from build123d import *

# Parameters (mm, degrees)
SKETCH1_R           = 1.5
BOSS_EXTRUDE1_DEPTH = 2.5
SKETCH2_R           = 2.5
BOSS_EXTRUDE2_DEPTH = 2
SKETCH3_R           = 1.49
CUT_EXTRUDE1_DEPTH  = 7


with BuildPart() as part:
    # Sketch1 → Boss-Extrude1 (new body)
    with BuildSketch(Plane(origin=(0, 0, 0), x_dir=(1, 0, 0), z_dir=(0, 1, 0))):
        with BuildLine():
            Line((-8.75, 14.25), (3.8, 14.25))
            Line((3.8, 14.25), (3.8, -14.25))
            Line((3.8, -14.25), (-8.75, -14.25))
            ThreePointArc((-8.75, -14.25), (-12.5, -18), (-8.75, -21.75))
            Line((-8.75, -21.75), (7.55, -21.75))
            ThreePointArc((7.55, -21.75), (10.201650429, -20.651650429), (11.3, -18))
            Line((11.3, -18), (11.3, 18))
            ThreePointArc((11.3, 18), (10.201650429, 20.651650429), (7.55, 21.75))
            Line((7.55, 21.75), (-8.75, 21.75))
            ThreePointArc((-8.75, 21.75), (-12.5, 18), (-8.75, 14.25))
        make_face()
        with Locations(Location((0, 18, 0), (0, 0, 270))):
            Circle(SKETCH1_R, mode=Mode.SUBTRACT)
        with Locations(Location((0, -18, 0), (0, 0, 270))):
            Circle(SKETCH1_R, mode=Mode.SUBTRACT)
    extrude(amount=BOSS_EXTRUDE1_DEPTH)

    # Sketch2 → Boss-Extrude2 (add)
    with BuildSketch(Plane.XZ):
        with Locations(Location((7.55, 0, 0), (0, 0, 90))):
            Circle(SKETCH2_R)
    extrude(amount=BOSS_EXTRUDE2_DEPTH)

    # Sketch3 → Cut-Extrude1 (cut)
    with BuildSketch(Plane.XZ.offset(2)):
        with Locations(Location((7.55, 0, 0), (0, 0, 270))):
            Circle(SKETCH3_R)
    extrude(amount=-CUT_EXTRUDE1_DEPTH, mode=Mode.SUBTRACT)


solid = part.part
Source: CAD feature listing. Evaluate the final solid. Frame: model axes, mm. A direction names the side the tool comes from. Give positions to 0.01 mm unless a question says otherwise; leave off trailing zeros. Order: outer loops, then holes, each group sorted by start corner. A loop starts at its lowest first (then second) coordinate and runs counter-clockwise, first axis right, second up. Notation, with made-up numbers: (73, -3) -> (112, -3) arc R27 ccw to (112, 19) -> close; hole circle Ø5 at (7, 19.25). An arc over 180 degrees is marked (long way). Write item = value, one per line.
Q1. Material intervals for line 1 (Z direction, x = -0.25, y = 2); line 2 (Z direction, x = -4, y = 1.85); line 3 (X direction, y = 1.05, z = 18), sorted ascending. Write a range as from..to.
Data:
line_1 = -21.75..-19.48, -16.52..-14.25, 14.25..16.52, 19.48..21.75
line_2 = -21.75..-14.25, 14.25..21.75
line_3 = -12.5..-1.5, 1.5..11.3
Q2. Pin query (flat end, axial travel): pin 1 (12 mm diameter, centred on x = -3.5, z = -5.5, fed in from -Y); pin 2 (12 mm diameter, centred on x = 2.5, z = -7, fed in from -Y); pin 3 (0.8 mm diameter, centred on y = 2, z = 7, fed in from -X). Return the tip coordinate at first contact, or that it passes through.
Data:
pin_1 = through
pin_2 = 0
pin_3 = 3.8
Q3. Pull-direction query (Z, two-part tool) for faces 1 (the face through (10.172, 1.232, 20.681)), 2 (the face through (10, -1, -0.5)), 3 (the face through (11.3, 1, 0)), 4 (the face through (0.07, 1.23, 16.5)); classes: released by +Z, released by -Z, zero draft, split by the parting line, or undercut.
Data:
face_1 = released by +Z
face_2 = split by the parting line
face_3 = zero draft
face_4 = undercut
Q4. Cut plane A-A, the plane z = 0. Output: boundary loops of the cut face in (x, y).
Data:
outline = (3.8, 0) -> (5.05, 0) -> (5.05, -2) -> (6.06, -2) -> (6.06, 2.5) -> (3.8, 2.5) -> close; (9.04, -2) -> (10.05, -2) -> (10.05, 0) -> (11.3, 0) -> (11.3, 2.5) -> (9.04, 2.5) -> close
Q5. Cut plane C-C, the plane x = 1. Output: boundary loops of the cut face in (y, z), and give its area (3 significant figures).
Data:
outline = (0, -21.75) -> (2.5, -21.75) -> (2.5, -19.12) -> (0, -19.12) -> close; (0, -16.88) -> (2.5, -16.88) -> (2.5, -14.25) -> (0, -14.25) -> close; (0, 14.25) -> (2.5, 14.25) -> (2.5, 16.88) -> (0, 16.88) -> close; (0, 19.12) -> (2.5, 19.12) -> (2.5, 21.75) -> (0, 21.75) -> close
area = 26.3 mm^2
Q6. Cut plane B-B, the plane x = -6.5. Output: boundary loops of the cut face in (y, z).
Data:
outline = (0, -21.75) -> (2.5, -21.75) -> (2.5, -14.25) -> (0, -14.25) -> close; (0, 14.25) -> (2.5, 14.25) -> (2.5, 21.75) -> (0, 21.75) -> close
Q7. Cut plane D-D, the plane y = 2.05. Output: boundary loops of the cut face in (x, z), and give its area (3 significant figures).
Data:
outline = (-8.75, -21.75) -> (7.55, -21.75) arc R3.75 ccw to (11.3, -18) -> (11.3, 18) arc R3.75 ccw to (7.55, 21.75) -> (-8.75, 21.75) arc R3.75 ccw to (-8.75, 14.25) -> (3.8, 14.25) -> (3.8, -14.25) -> (-8.75, -14.25) arc R3.75 ccw to start; hole circle Ø3 at (0, -18); hole circle Ø3 at (0, 18); hole circle Ø2.98 at (7.55, 0)
area = 532 mm^2
Q8. Set-up query: faces 5 (the face through (-1, 1, 21.75)), 6 (the face through (-3, 1, -14.25)). Return all of +Z, -Z, +X, -X, +Y, -Y with unobstructed straight access to the full face (end or side cutting, diameter ignored); none if empty.
Data:
face_5 = +Z, +X, -X, +Y, -Y
face_6 = -X, +Y, -Y
